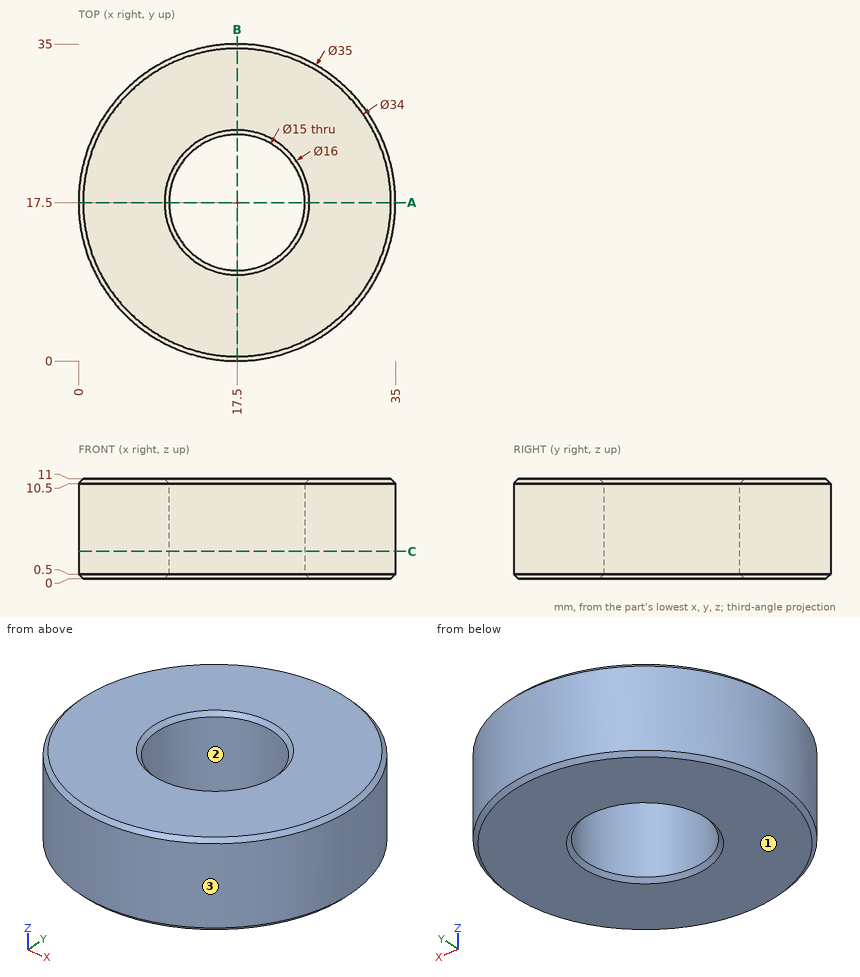
The figure shows three views and two pictorial views of one solid part (mm, origin at its lowest corner). Answer the questions. Give positions to 0.01 mm unless a question says otherwise; leave off trailing zeros. Loops run counter-clockwise (first coordinate to the right, second up) from the corner with the lowest first, then second, coordinate; pieces in that order, holes last. Notation, with made-up numbers: (25, -8) -> (60, -8) arc R23 cw to (60, 23) -> close; hole circle Ø2 at (75, 33). An arc over 180 degrees is marked (long way). Use CSV: the item, a comma, the result in double quotes.
1. The part is cut by section C-C (z = 3). Write down the section's boundary in (x, y).
Found:
outline,"circle Ø35 at (17.5, 17.5); hole circle Ø15 at (17.5, 17.5)"
2. The mould has two halves that part along Y. Classify the marked faces 1, 2 and 3: +Y half, -Y half, draft (parallel to the pull), parting line (faces both ways), or undercut.
Found:
face 1,"draft"
face 2,"undercut"
face 3,"parting line"
3. The part is cut by section A-A (y = 17.5). Write down the section's boundary in (x, z), then the cut area to 3 significant figures.
Found:
outline,"(0, 0.5) -> (0.5, 0) -> (9.5, 0) -> (10, 0.5) -> (10, 10.5) -> (9.5, 11) -> (0.5, 11) -> (0, 10.5) -> close; (25, 0.5) -> (25.5, 0) -> (34.5, 0) -> (35, 0.5) -> (35, 10.5) -> (34.5, 11) -> (25.5, 11) -> (25, 10.5) -> close"
area,"219 mm^2"
4. Straight lines are drawn through the part: line 1 (Y direction, x = 17.5, z = 6.75); line 2 (Y direction, x = 24, z = 6.25); line 3 (X direction, y = 12, z = 1.5). For each, find the intervals that lie inside material, in ascending order.
Found:
line 1,"0 to 10, 25 to 35"
line 2,"1.25 to 13.76, 21.24 to 33.75"
line 3,"0.89 to 12.4, 22.6 to 34.11"
5. Flat-ended cylindrical pins translate along their axes: pin 1 Ø6 at (x, z) = (20, 5.5) entering from +Y; pin 2 Ø5 at (x, z) = (26, 9.5) entering from +Y; pin 3 Ø4 at (y, z) = (20, 2) entering from -X; pin 4 Ø3 at (y, z) = (6.5, 4) entering from -X. Find the tip coordinate at first contact, or state that the pin passes through.
Found:
pin 1,"y = 35"
pin 2,"y = 33.94"
pin 3,"x = 0.01"
pin 4,"x = 2.8"
